Read the model definition and answer for the solid it produces. Units are mm, in the model's axes. A direction names the side the tool comes from. Give positions to 0.01 mm unless a question says otherwise; leave off trailing zeros. Write each loop counter-clockwise with the first axis right and the second up, starting at its lowest first coordinate (ties: lowest second). Pieces come first, ordered by that corner, then holes. Notation, with made-up numbers: M 52,47 L 98,47 A28 ccw 98,83 Z; hole C -13.75,-23.5 d11. An arc over 180 degrees is marked long. Put each result on its own line as item: value.
from build123d import *

# Parameters (mm, degrees)
SKETCH1_W           = 35
SKETCH1_H           = 120
BOSS_EXTRUDE1_DEPTH = 7.5
BOSS_EXTRUDE2_DEPTH = 20
SKETCH4_R           = 1.4
CUT_EXTRUDE2_DEPTH  = 12
SKETCH5_R           = 2.5
SKETCH5_R_2         = 1.4
CUT_EXTRUDE3_DEPTH  = 2.5


with BuildPart() as part:
    # Sketch1 → Boss-Extrude1 (new body)
    with BuildSketch(Plane(origin=(0, 0, 0), x_dir=(1, 0, 0), z_dir=(0, 1, 0))):
        with Locations((-17.5, 0)):
            Rectangle(SKETCH1_W, SKETCH1_H)
    extrude(amount=BOSS_EXTRUDE1_DEPTH)

    # Sketch2 → Boss-Extrude2 (add)
    with BuildSketch(Plane(origin=(0, 7.5, 0), x_dir=(1, 0, 0), z_dir=(0, 1, 0))):
        Polygon((0, 5.05), (-32.5, 5.05), (-32.5, 60), (-35, 60), (-35, 2.55), (0, 2.55), align=None)
        Polygon((0, -5.05), (0, -2.55), (-35, -2.55), (-35, -60), (-32.5, -60), (-32.5, -5.05), align=None)
    extrude(amount=BOSS_EXTRUDE2_DEPTH)

    # Sketch4 → Cut-Extrude2 (cut)
    with BuildSketch(Plane.XY.offset(5.05)):
        with Locations(Location((-5, 25, 0), (0, 0, 180))):
            Circle(SKETCH4_R)
        with Locations(Location((-20, 25, 0), (0, 0, 180))):
            Circle(SKETCH4_R)
        with Locations(Location((-5, 15, 0), (0, 0, 180))):
            Circle(SKETCH4_R)
        with Locations(Location((-20, 15, 0), (0, 0, 180))):
            Circle(SKETCH4_R)
    extrude(amount=-CUT_EXTRUDE2_DEPTH, mode=Mode.SUBTRACT)

    # Sketch5 → Cut-Extrude3 (cut)
    with BuildSketch(Plane(origin=(-32.5, 0, 0), x_dir=(0, 0, -1), z_dir=(1, 0, 0))):
        with Locations((-48, 17.5)):
            Circle(SKETCH5_R)
        with Locations((-48, 24.5)):
            Circle(SKETCH5_R_2)
        with Locations((-55, 17.5)):
            Circle(SKETCH5_R_2)
        with Locations(Location((-48, 10.5, 0), (0, 0, 180))):
            Circle(SKETCH5_R_2)
        with Locations(Location((-41, 17.5, 0), (0, 0, 180))):
            Circle(SKETCH5_R_2)
        with Locations((41, 17.5)):
            Circle(SKETCH5_R_2)
        with Locations((48, 10.5)):
            Circle(SKETCH5_R_2)
        with Locations(Location((55, 17.5, 0), (0, 0, 180))):
            Circle(SKETCH5_R_2)
        with Locations(Location((48, 24.5, 0), (0, 0, 180))):
            Circle(SKETCH5_R_2)
        with Locations(Location((48, 17.5, 0), (0, 0, 180))):
            Circle(SKETCH5_R)
    extrude(amount=-CUT_EXTRUDE3_DEPTH, mode=Mode.SUBTRACT)


solid = part.part
(1) Section C-C on x = -24.5 is taken. Determine the outline of the cut face in (y, z).
Result:
outline: M 0,-60 L 7.5,-60 L 7.5,-5.05 L 27.5,-5.05 L 27.5,-2.55 L 7.5,-2.55 L 7.5,2.55 L 27.5,2.55 L 27.5,5.05 L 7.5,5.05 L 7.5,60 L 0,60 Z
(2) For a pull along X with two mould halves and no side action, classify faces 1 (the face through (-33.73, 25.74, -47.35)), 2 (the face through (0, 6, 0)), 3 (the face through (-5.75, 13.82, 3.82)) as +X half, -X half, draft (parallel to the pull), parting line (faces both ways), or undercut.
Result:
face 1: draft
face 2: +X half
face 3: undercut
(3) Given pin 1 Ø4.5 at (x, y) = (-20, 25) entering from -Z; pin 2 Ø16 at (x, z) = (-22, 36.5) entering from +Y; pin 3 Ø1.7 at (y, z) = (24.5, -48) entering from +X; pin 4 Ø4.5 at (y, z) = (10.5, -48) entering from +X, each flat-ended and moving along its own axis, determine where each tip first touches the part or whether it passes through.
Result:
pin 1: stops at z = -5.05
pin 2: stops at y = 7.5
pin 3: passes through
pin 4: stops at x = -32.5
(4) Section B-B on z = 48 is taken. Determine the outline of the cut face in (x, y), and give its area (3 significant figures).
Result:
outline: M -35,0 L 0,0 L 0,7.5 L -32.5,7.5 L -32.5,9.1 L -35,9.1 Z; M -35,11.9 L -32.5,11.9 L -32.5,15 L -35,15 Z; M -35,20 L -32.5,20 L -32.5,23.1 L -35,23.1 Z; M -35,25.9 L -32.5,25.9 L -32.5,27.5 L -35,27.5 Z
area: 286 mm²
(5) Which of the six approach directions +Z, -Z, +X, -X, +Y, -Y give full straight-line access (tool end or side, diameter ignored) to faces 4 (the face through (-33.73, 18.46, -45.69)), 5 (the face through (-17, 17, 2.55)), 6 (the face through (-32.5, 17, -32))?
Result:
face 4: +X, -X
face 5: +X, -X, +Y
face 6: -Z, +X, +Y
(6) Section A-A on z = -55 is taken. Determine the outline of the cut face in (x, y), and give its area (4 significant figures).
Result:
outline: M -35,0 L 0,0 L 0,7.5 L -32.5,7.5 L -32.5,16.1 L -35,16.1 Z; M -35,18.9 L -32.5,18.9 L -32.5,27.5 L -35,27.5 Z
area: 305.5 mm²
(7) Section D-D on y = 17.5 is taken. Give the number of separate pieces and of enclosed holes in the cut face, and give its area (3 significant figures).
Result:
separate pieces: 8
enclosed holes: 0
area: 397 mm²
(8) Straight lines are drawn through the part: line 1 along Y through (x, z) = (-5, 3.4); line 2 along Y through (x, z) = (-33.4, -48); line 3 along X through (y, z) = (15, -4.5). For each, find the intervals that lie inside material, in ascending order. Write a range as from..to.
Result:
line 1: y = 0..13.6, 16.4..23.6, 26.4..27.5
line 2: y = 0..9.1, 11.9..15, 20..23.1, 25.9..27.5
line 3: x = -35..-21.4, -18.6..-6.4, -3.6..0
